The model under review builds one solid part; all positions refer to its coordinate system, in mm. A direction names the side the tool comes from. Coordinates: 2 decimals unless noted, no trailing zeros. Write each loop counter-clockwise with the first axis right and the second up, starting at its lowest first coordinate (ties: lowest second). Pieces come first, ordered by that corner, then holes.
```python
from build123d import *

# Parameters (mm, degrees)
F0_W         = 112.5
F0_H         = 7
F0_R         = 1.5
F0_W_2       = 135
F0_W_3       = 2
F0_H_2       = 2
F0_H_3       = 9
F0_W_4       = 5.5
F0_R_2       = 1
F0_W_5       = 2.2
F0_H_4       = 3.5
F0_H_5       = 9.5
F1_DEPTH     = 1.5
F2_R         = 1
F3_T1_DEPTH  = 6.5
F3_T4_ANGLE  = 90
F3_T6_ANGLE  = 90
F3_T8_ANGLE  = 90
F3_T10_ANGLE = 90
F4_SIZE      = 1
F5_SIZE      = 1
F6_SIZE      = 1.49999


# Not quite as in the source:
# - a fillet or chamfer that OpenCascade refuses, or shapes differently, is made with other operations: its cross-section is extruded or revolved along the edge and cut away or added
# - a fillet or chamfer is up to 0.001 mm smaller than in the source, because OpenCascade refuses the exact size
# - a feature names something its author has since deleted; it is built from what else it names


with BuildPart() as f1:
    # F0 (on Top) → F1 (new body)
    with BuildSketch(Plane.XY):
        Polygon((54.1, 8.075), (54.1, 17.075), (52.1, 17.075), (52.1, 10.075), (-60.4, 10.075), (-60.4, 8.075), (-54.9, 8.075), align=None)
        Polygon((-60.4, 17.075), (52.1, 17.075), (52.1, 19.075), (-62.4, 19.075), (-62.4, 10.075), (-60.4, 10.075), align=None)
        with Locations((-4.15, 13.575)):
            Rectangle(F0_W, F0_H)
        with Locations((-56.4, 14.575)):
            Circle(F0_R, mode=Mode.SUBTRACT)
        with Locations((5.1, 14.575)):
            Circle(F0_R, mode=Mode.SUBTRACT)
        Polygon((54.1, 17.075), (70.6, 17.075), (70.6, 13.575), (72.6, 13.575), (72.6, 19.075), (52.1, 19.075), (52.1, 17.075), align=None)
        Polygon((70.6, 13.575), (70.6, 17.075), (54.1, 17.075), (54.1, 8.075), (-54.9, 8.075), (-54.9, -0.925), (-54.9, -2.925), (-54.9, -21.425), (70.6, -21.425), (70.6, 4.575), align=None)
        with BuildLine():
            Line((56.6, 4.575), (56.6, -15.925))
            ThreePointArc((56.6, -15.925), (55.7213203436, -18.0463203436), (53.6, -18.925))
            Line((53.6, -18.925), (-45.4, -18.925))
            ThreePointArc((-45.4, -18.925), (-47.5213203436, -18.0463203436), (-48.4, -15.925))
            Line((-48.4, -15.925), (-48.4, 4.575))
            ThreePointArc((-48.4, 4.575), (-48.1071067812, 5.2821067812), (-47.4, 5.575))
            Line((-47.4, 5.575), (55.6, 5.575))
            ThreePointArc((55.6, 5.575), (56.3071067812, 5.2821067812), (56.6, 4.575))
        make_face(mode=Mode.SUBTRACT)
        with Locations((64.6, -12.425)):
            Circle(F0_R, mode=Mode.SUBTRACT)
        with Locations((64.6, -4.425)):
            Circle(F0_R, mode=Mode.SUBTRACT)
        with Locations((64.6, 3.575)):
            Circle(F0_R, mode=Mode.SUBTRACT)
        with Locations((61.6, 9.075)):
            Circle(F0_R, mode=Mode.SUBTRACT)
        Polygon((72.6, 4.575), (70.6, 4.575), (70.6, -21.425), (-54.9, -21.425), (-56.55, -21.425), (-58.75, -21.425), (-60.4, -21.425), (-60.4, -2.925), (-62.4, -2.925), (-62.4, -23.425), (72.6, -23.425), align=None)
        with Locations((5.1, -26.925)):
            Rectangle(F0_W_2, F0_H)
        with Locations((-56.4, -25.925)):
            Circle(F0_R, mode=Mode.SUBTRACT)
        with Locations((5.1, -25.925)):
            Circle(F0_R, mode=Mode.SUBTRACT)
        with Locations((66.6, -25.925)):
            Circle(F0_R, mode=Mode.SUBTRACT)
        with Locations((-61.4, 9.075)):
            Rectangle(F0_W_3, F0_H_2)
        with Locations((-61.4, 3.575)):
            Rectangle(F0_W_3, F0_H_3)
        with Locations((-61.4, -1.925)):
            Rectangle(F0_W_3, F0_H_2)
        with Locations((-57.65, 3.575)):
            Rectangle(F0_W_4, F0_H_3)
        with Locations((-57.65, 3.575)):
            Circle(F0_R_2, mode=Mode.SUBTRACT)
        Polygon((-54.9, -2.925), (-54.9, -0.925), (-60.4, -0.925), (-60.4, -2.925), (-58.75, -2.925), (-56.55, -2.925), align=None)
        with Locations((-57.65, -4.675)):
            Rectangle(F0_W_5, F0_H_4)
        Polygon((-56.55, -21.425), (-54.9, -21.425), (-54.9, -2.925), (-56.55, -2.925), (-56.55, -6.425), (-56.55, -11.925), align=None)
        Polygon((-58.75, -2.925), (-60.4, -2.925), (-60.4, -21.425), (-58.75, -21.425), (-58.75, -11.925), (-58.75, -6.425), align=None)
        with Locations((-57.65, -16.675)):
            Rectangle(F0_W_5, F0_H_5)
    extrude(amount=F1_DEPTH)

    # F2
    f2_edges = [f1.edges().sort_by_distance(p)[0] for p in [
        (-62.4, -5.675, 1.5),
        (5.1, 19.075, 1.5),
        (72.6, 16.325, 1.5),
        (72.6, -12.925, 1.5),
        (5.1, -30.425, 1.5),
    ]]
    fillet(f2_edges, radius=F2_R)

    # F3: fillet of radius 2 on 4 edges, made by hand

    # F3_s2 → F3_t1 (cut)
    with BuildSketch(Plane.XY.offset(-5)):
        with BuildLine():
            ThreePointArc((-60.4, 19.075), (-61.8142135624, 18.4892135624), (-62.4, 17.075))
            Line((-62.4, 17.075), (-62.4, 19.075))
            Line((-62.4, 19.075), (-60.4, 19.075))
        make_face()
        with BuildLine():
            ThreePointArc((72.6, 17.075), (72.0142135624, 18.4892135624), (70.6, 19.075))
            Line((70.6, 19.075), (72.6, 19.075))
            Line((72.6, 19.075), (72.6, 17.075))
        make_face()
        with BuildLine():
            ThreePointArc((70.6, -30.425), (72.0142135624, -29.8392135624), (72.6, -28.425))
            Line((72.6, -28.425), (72.6, -30.425))
            Line((72.6, -30.425), (70.6, -30.425))
        make_face()
        with BuildLine():
            ThreePointArc((-62.4, -28.425), (-61.8142135624, -29.8392135624), (-60.4, -30.425))
            Line((-60.4, -30.425), (-62.4, -30.425))
            Line((-62.4, -30.425), (-62.4, -28.425))
        make_face()
    extrude(amount=F3_T1_DEPTH, mode=Mode.SUBTRACT)

    # F3_s3 → F3_t4 (revolve, cut)
    with BuildSketch(Plane.XZ.offset(28.425)):
        with BuildLine():
            ThreePointArc((-61.4, 1.5), (-62.1071067812, 1.2071067812), (-62.4, 0.5))
            Line((-62.4, 0.5), (-62.4, 1.5))
            Line((-62.4, 1.5), (-61.4, 1.5))
        make_face()
    revolve(axis=Axis((-60.4, -28.425, 1.5), (0, 0, 1)), revolution_arc=F3_T4_ANGLE, mode=Mode.SUBTRACT)

    # F3_s5 → F3_t6 (revolve, cut)
    with BuildSketch(Plane.YZ.offset(70.6)):
        with BuildLine():
            ThreePointArc((-29.425, 1.5), (-30.1321067812, 1.2071067812), (-30.425, 0.5))
            Line((-30.425, 0.5), (-30.425, 1.5))
            Line((-30.425, 1.5), (-29.425, 1.5))
        make_face()
    revolve(axis=Axis((70.6, -28.425, 1.5), (0, 0, 1)), revolution_arc=F3_T6_ANGLE, mode=Mode.SUBTRACT)

    # F3_s7 → F3_t8 (revolve, cut)
    with BuildSketch(Plane.XZ.offset(-17.075)):
        with BuildLine():
            ThreePointArc((71.6, 1.5), (72.3071067812, 1.2071067812), (72.6, 0.5))
            Line((72.6, 0.5), (72.6, 1.5))
            Line((72.6, 1.5), (71.6, 1.5))
        make_face()
    revolve(axis=Axis((70.6, 17.075, 1.5), (0, 0, 1)), revolution_arc=F3_T8_ANGLE, mode=Mode.SUBTRACT)

    # F3_s9 → F3_t10 (revolve, cut)
    with BuildSketch(Plane.YZ.offset(-60.4)):
        with BuildLine():
            ThreePointArc((18.075, 1.5), (18.7821067812, 1.2071067812), (19.075, 0.5))
            Line((19.075, 0.5), (19.075, 1.5))
            Line((19.075, 1.5), (18.075, 1.5))
        make_face()
    revolve(axis=Axis((-60.4, 17.075, 1.5), (0, 0, 1)), revolution_arc=F3_T10_ANGLE, mode=Mode.SUBTRACT)

    # F4
    f4_edges = [f1.edges().sort_by_distance(p)[0] for p in [
        (4.1, 5.575, 1.5),
        (55.72132, -18.04632, 1.5),
        (56.6, -5.675, 1.5),
        (56.307107, 5.282107, 1.5),
    ]]
    chamfer(f4_edges, length=F4_SIZE)

    # F5
    f5_edges = [f1.edges().sort_by_distance(p)[0] for p in [
        (63.1, 3.575, 1.5),
        (63.1, -4.425, 1.5),
        (63.1, -12.425, 1.5),
    ]]
    chamfer(f5_edges, length=F5_SIZE)

    # F6 (size 1.5 in the source; OpenCascade refuses exactly that, so slightly less here)
    f6_edges = [f1.edges().sort_by_distance(p)[0] for p in [
        (3.6, 14.575, 1.5),
        (60.1, 9.075, 1.5),
        (65.1, -25.925, 1.5),
        (3.6, -25.925, 1.5),
        (-57.9, -25.925, 1.5),
        (-57.9, 14.575, 1.5),
    ]]
    chamfer(f6_edges, length=F6_SIZE)


solid = f1.part
```
Item 1: Machinability: for faces 1 (the face through (-47.5, -18.07, 0.25)), 2 (the face through (55.94, -18.21, 0.77)), which of the approach directions +Z, -Z, +X, -X, +Y, -Y give a long, thin tool a straight path to every point of the face, cutting with its end or side? Answer none if there is none.
Solved:
face 1: +Z, -Z
face 2: +Z
Item 2: To check wall thickness, follow line 1 along Y through (x, z) = (64.6, 0.2) (3 decimals); line 2 along X through (y, z) = (-8.5, 0.2); line 3 along X through (y, z) = (-5.5, 1.35). State the ranges of each line that lie inside material, in increasing order.
Solved:
line 1: y = -30.425 to -13.925, -10.925 to -5.925, -2.925 to 2.075, 5.075 to 19.075
line 2: x = -62.4 to -58.75, -56.55 to -48.4, 56.6 to 72.6
line 3: x = -61.93 to -49.25, 57.45 to 62.51, 66.69 to 72.13
Item 3: For pin 1 (0.8 mm diameter, centred on x = -58, z = 1, fed in from +Y); pin 2 (3.5 mm diameter, centred on x = 64.6, y = -4.425, fed in from +Z), all flat-tipped, find the tip position at first contact; note any pin that passes through.
Solved:
pin 1: stops at y = 19.07
pin 2: stops at z = 0.75
Item 4: Mouldability with a two-part tool opening along X and no side actions: class faces 3 (the face through (4, -21, 1.5)), 4 (the face through (65.986, -13, 0.246)) as pulls with the +X half, pulls with the -X half, needs draft (parallel to the pull), parting line crosses it, or undercut.
Solved:
face 3: needs draft
face 4: undercut
Item 5: Take a section at A-A, the plane x = 34. Write out the cut boundary in (y, z) (3 decimals), plus the area to 3 significant figures.
Solved:
outline: (-30.425, 0) - (-18.925, 0) - (-18.925, 0.5) - (-19.925, 1.5) - (-29.425, 1.5) arc R1 ccw to (-30.425, 0.5) - close; (5.575, 0) - (19.075, 0) - (19.075, 0.5) arc R1 ccw to (18.075, 1.5) - (6.575, 1.5) - (5.575, 0.5) - close
area: 36.1 mm2
Item 6: Take a section at B-B, the plane x = 5.1. Count the separate pieces of the cut face and the enclosed holes in it, plus the area to 3 significant figures.
Solved:
separate pieces: 4
enclosed holes: 0
area: 22.6 mm2
